Part model, mm, in its own coordinate system. A direction names the side the tool comes from. Coordinates: 2 decimals unless noted, no trailing zeros. Loops run counter-clockwise (first coordinate to the right, second up) from the corner with the lowest first, then second, coordinate; pieces in that order, holes last. Notation, with made-up numbers: M -26,56 L -2,56 A14 ccw -2,61 Z; hole C 66.5,-3 d10. An arc over 180 degrees is marked long. Answer as a JSON object with one key per item and string values. Group by question number.
1. Drop flat-ended pins along their axis: pin 1 Ø2 at (y, z) = (-0.5, 14.5) entering from -X; pin 2 Ø14 at (y, z) = (-20, 1.6) entering from +X; pin 3 Ø2 at (y, z) = (1.5, 14.5) entering from +X; pin 4 Ø4 at (y, z) = (5, 9.5) entering from -X. Give the stop position or say it passes through.
2. Saw through at D-D on x = 15.5. Write the cut outline in (y, z).
3. Saw through at B-B on x = -3. Write the cut outline in (y, z).
4. Saw through at A-A on y = 2.5. Write the cut outline in (x, z), then the cut area to 3 significant figures.
5. Saw through at C-C on y = -19. Write the cut outline in (x, z), then the cut area to 3 significant figures.
6. Drill centre lines: L1, parallel to Y at x = 0.75, z = 1.6; L2, parallel to Z at x = 4, y = -2.5. Where is each one in solid material? Low to high.
7. Mould opens along X. For faces 6 (the face through (0, 0, 12)), 7 (the face through (-29.3, 7.5, 9.3)) say: released by +X, released by -X, zero draft, split by the parting line, or undercut.
8. 3-axis set-ups, long thin cutter, end or side, ignore diameter. For faces 1 (the face through (14, 0, -10)), 2 (the face through (0, -15, -10)), 3 (the face through (31, 7.5, 6)), 4 (the face through (-9.436, 0, 14)), 5 (the face through (0, 0, -8)): which of +Z, -Z, +X, -X, +Y, -Y reach the whole face in a straight line?
from build123d import *

# Parameters (mm, degrees)
F1_DEPTH = 7.5
F3_DEPTH = 7.5


with BuildPart() as f1:
    # F0 (on Front) → F1 (new body, symmetric)
    with BuildSketch(Plane.XZ):
        with BuildLine():
            Line((9.436439, 16), (9.436439, 12))
            Line((9.436439, 12), (-9.436439, 12))
            Line((-9.436439, 12), (-9.436439, 16))
            Line((-9.436439, 16), (-11.236439, 16))
            Line((-11.236439, 16), (-11.236439, 12))
            ThreePointArc((-11.236439, 12), (-32.774976, 6.264762), (-20, -12))
            Line((-20, -12), (20, -12))
            ThreePointArc((20, -12), (32.774976, 6.264762), (11.236439, 12))
            Line((11.236439, 12), (11.236439, 16))
            Line((11.236439, 16), (9.436439, 16))
        make_face()
        with BuildLine():
            Line((-12, 10), (12, 10))
            ThreePointArc((12, 10), (30.77033, 5.908132), (20, -10))
            Line((20, -10), (-20, -10))
            ThreePointArc((-20, -10), (-30.77033, 5.908132), (-12, 10))
        make_face(mode=Mode.SUBTRACT)
    extrude(amount=F1_DEPTH, both=True)

    # F2 (on Right) → F3 (join, symmetric)
    with BuildSketch(Plane.YZ):
        with BuildLine():
            Line((-7.5, -10), (7.5, -10))
            Line((7.5, -10), (7.5, -12))
            Line((7.5, -12), (20, -12))
            ThreePointArc((20, -12), (32.231108, 7.546427), (9.304206, 10))
            Line((9.304206, 10), (8.7, 12))
            Line((8.7, 12), (7.5, 12))
            Line((7.5, 12), (7.5, 10))
            Line((7.5, 10), (-7.5, 10))
            Line((-7.5, 10), (-7.5, 12))
            Line((-7.5, 12), (-8.7, 12))
            Line((-8.7, 12), (-9.304206, 10))
            ThreePointArc((-9.304206, 10), (-32.231108, 7.546427), (-20, -12))
            Line((-20, -12), (-7.5, -12))
            Line((-7.5, -12), (-7.5, -10))
        make_face()
        with BuildLine():
            Line((-10.7, -10), (-20, -10))
            ThreePointArc((-20, -10), (-30.217632, 7.091812), (-10.325291, 8))
            Line((-10.325291, 8), (10.325291, 8))
            ThreePointArc((10.325291, 8), (30.217632, 7.091812), (20, -10))
            Line((20, -10), (10.7, -10))
            Line((10.7, -10), (8.7, -8))
            Line((8.7, -8), (-8.7, -8))
            Line((-8.7, -8), (-10.7, -10))
        make_face(mode=Mode.SUBTRACT)
    extrude(amount=F3_DEPTH, both=True)


solid = f1.part
Outcome:
{
 "1": {"pin 1": "stops at x = -26.58", "pin 2": "passes through", "pin 3": "stops at x = 26.58", "pin 4": "stops at x = -32.25"},
 "2": {"outline": "M -7.5,-12 L 7.5,-12 L 7.5,-10 L -7.5,-10 Z; M -7.5,12.29 L 7.5,12.29 L 7.5,14.43 L -7.5,14.43 Z"},
 "3": {"outline": "M -20,-12 L 20,-12 A13.6 ccw long 9.3,10 L 8.7,12 L -8.7,12 L -9.3,10 A13.6 ccw long Z; hole M -20,-10 L -10.7,-10 L -8.7,-8 L 8.7,-8 L 10.7,-10 L 20,-10 A11.6 ccw long 10.33,8 L -10.33,8 A11.6 ccw long Z"},
 "4": {"outline": "M -20,-12 L 20,-12 A13.6 ccw long 11.24,12 L 11.24,16 L 9.44,16 L 9.44,12 L -9.44,12 L -9.44,16 L -11.24,16 L -11.24,12 A13.6 ccw long Z; hole M -20,-10 L -7.5,-10 L -7.5,-8 L 7.5,-8 L 7.5,-10 L 20,-10 A11.6 ccw long 12,10 L 7.5,10 L 7.5,8 L -7.5,8 L -7.5,10 L -12,10 A11.6 ccw long Z", "area": "396 mm²"},
 "5": {"outline": "M -7.5,-12 L 7.5,-12 L 7.5,-10 L -7.5,-10 Z; M -7.5,13.16 L 7.5,13.16 L 7.5,15.16 L -7.5,15.16 Z", "area": "60.1 mm²"},
 "6": {"L1": "y = -33.6 to -31.6, 31.6 to 33.6", "L2": "z = -12 to -8, 8 to 12"},
 "7": {"face 6": "undercut", "face 7": "zero draft"},
 "8": {"face 1": "+Y, -Y", "face 2": "+X, -X", "face 3": "+Z, -Z, +X, +Y", "face 4": "+Z, +Y, -Y", "face 5": "none"}
}
